from build123d import *

# Parameters (mm, degrees)
SKETCH_1_W          = 553
SKETCH_1_H          = 333
EXTRUDE_1_DEPTH     = 56
FILLET_1_SIZE       = 40
FILLET_1_SIZE_2     = 150
SKETCH_2_W          = 526
SKETCH_2_H          = 298
CUT_EXTRUDE_1_DEPTH = 1
SKETCH_3_W          = 90
SKETCH_3_H          = 7.88506372
EXTRUDE_2_DEPTH     = 3


with BuildPart() as part:
    # Эскиз1 → Бобышка-Вытянуть1 (new body)
    with BuildSketch(Plane.XY):
        with Locations((219.863599641, -140.079802513)):
            Rectangle(SKETCH_1_W, SKETCH_1_H)
    extrude(amount=-EXTRUDE_1_DEPTH)

    # Скругление1
    # an asymmetric fillet: 150, 40 mm, written as the material it takes off along each edge
    with BuildSketch(Plane(origin=(496.363599641, -306.579802513, -56), x_dir=(0, 0, 1), z_dir=(-1, 0, 0)), Plane(origin=(-56.636400359, 26.420197487, -56), x_dir=(0, 0, 1), z_dir=(1, 0, 0))) as fillet_1_piece_1:
        with BuildLine():
            Bezier((FILLET_1_SIZE, 0), (0, 0), (0, FILLET_1_SIZE_2), weights=[1, 0.707106781, 1])
            Line((0, FILLET_1_SIZE_2), (-3, 150))
            Line((-3, 150), (-3, -3))
            Line((-3, -3), (40, -3))
            Line((40, -3), (FILLET_1_SIZE, 0))
        make_face()
    extrude(amount=553, mode=Mode.SUBTRACT)
    with BuildSketch(Plane(origin=(-56.636400359, -306.579802513, -56), x_dir=(0, 0, 1), z_dir=(0, 1, 0)), Plane(origin=(496.363599641, 26.420197487, -56), x_dir=(0, 0, 1), z_dir=(0, -1, 0))) as fillet_1_piece_2:
        with BuildLine():
            Bezier((FILLET_1_SIZE, 0), (0, 0), (0, FILLET_1_SIZE_2), weights=[1, 0.707106781, 1])
            Line((0, FILLET_1_SIZE_2), (-3, 150))
            Line((-3, 150), (-3, -3))
            Line((-3, -3), (40, -3))
            Line((40, -3), (FILLET_1_SIZE, 0))
        make_face()
    extrude(amount=333, mode=Mode.SUBTRACT)
    with BuildSketch(Plane(origin=(496.363599641, 26.420197487, -56), x_dir=(0, 0, 1), z_dir=(0, -1, 0))) as fillet_1_piece_3a_section:
        with BuildLine():
            Bezier((FILLET_1_SIZE, 0), (0, 0), (0, FILLET_1_SIZE_2), weights=[1, 0.707106781, 1])
            Line((0, FILLET_1_SIZE_2), (-3, 150))
            Line((-3, 150), (-3, -3))
            Line((-3, -3), (40, -3))
            Line((40, -3), (FILLET_1_SIZE, 0))
        make_face()
    fillet_1_piece_3a = extrude(amount=708, mode=Mode.PRIVATE)
    fillet_1_piece_3a = split(fillet_1_piece_3a, bisect_by=Plane(origin=(455.274079594, -306.579802513, -48.919820082), z_dir=(0, -1, 0)), keep=Keep.TOP, mode=Mode.PRIVATE)
    with BuildSketch(Plane(origin=(871.363599641, -306.579802513, -56), x_dir=(0, 0, 1), z_dir=(-1, 0, 0))) as fillet_1_piece_3b_section:
        with BuildLine():
            Bezier((FILLET_1_SIZE, 0), (0, 0), (0, FILLET_1_SIZE_2), weights=[1, 0.707106781, 1])
            Line((0, FILLET_1_SIZE_2), (-3, 150))
            Line((-3, 150), (-3, -3))
            Line((-3, -3), (40, -3))
            Line((40, -3), (FILLET_1_SIZE, 0))
        make_face()
    fillet_1_piece_3b = extrude(amount=928, mode=Mode.PRIVATE)
    fillet_1_piece_3b = split(fillet_1_piece_3b, bisect_by=Plane(origin=(496.363599641, -265.490295874, -48.919826396), z_dir=(1, 0, 0)), keep=Keep.TOP, mode=Mode.PRIVATE)
    fillet_1_piece_3 = fillet_1_piece_3a & fillet_1_piece_3b
    add(fillet_1_piece_3, mode=Mode.SUBTRACT)
    with BuildSketch(Plane(origin=(496.363599641, -306.579802513, -56), x_dir=(0, 0, 1), z_dir=(-1, 0, 0))) as fillet_1_piece_4a_section:
        with BuildLine():
            Bezier((FILLET_1_SIZE, 0), (0, 0), (0, FILLET_1_SIZE_2), weights=[1, 0.707106781, 1])
            Line((0, FILLET_1_SIZE_2), (-3, 150))
            Line((-3, 150), (-3, -3))
            Line((-3, -3), (40, -3))
            Line((40, -3), (FILLET_1_SIZE, 0))
        make_face()
    fillet_1_piece_4a = extrude(amount=928, mode=Mode.PRIVATE)
    fillet_1_piece_4a = split(fillet_1_piece_4a, bisect_by=Plane(origin=(-56.636400359, -265.49028305, -48.919819953), z_dir=(-1, 0, 0)), keep=Keep.TOP, mode=Mode.PRIVATE)
    with BuildSketch(Plane(origin=(-56.636400359, -681.579802513, -56), x_dir=(0, 0, 1), z_dir=(0, 1, 0))) as fillet_1_piece_4b_section:
        with BuildLine():
            Bezier((FILLET_1_SIZE, 0), (0, 0), (0, FILLET_1_SIZE_2), weights=[1, 0.707106781, 1])
            Line((0, FILLET_1_SIZE_2), (-3, 150))
            Line((-3, 150), (-3, -3))
            Line((-3, -3), (40, -3))
            Line((40, -3), (FILLET_1_SIZE, 0))
        make_face()
    fillet_1_piece_4b = extrude(amount=708, mode=Mode.PRIVATE)
    fillet_1_piece_4b = split(fillet_1_piece_4b, bisect_by=Plane(origin=(-15.546893136, -306.579802513, -48.919826525), z_dir=(0, -1, 0)), keep=Keep.TOP, mode=Mode.PRIVATE)
    fillet_1_piece_4 = fillet_1_piece_4a & fillet_1_piece_4b
    add(fillet_1_piece_4, mode=Mode.SUBTRACT)
    with BuildSketch(Plane(origin=(-431.636400359, 26.420197487, -56), x_dir=(0, 0, 1), z_dir=(1, 0, 0))) as fillet_1_piece_5a_section:
        with BuildLine():
            Bezier((FILLET_1_SIZE, 0), (0, 0), (0, FILLET_1_SIZE_2), weights=[1, 0.707106781, 1])
            Line((0, FILLET_1_SIZE_2), (-3, 150))
            Line((-3, 150), (-3, -3))
            Line((-3, -3), (40, -3))
            Line((40, -3), (FILLET_1_SIZE, 0))
        make_face()
    fillet_1_piece_5a = extrude(amount=928, mode=Mode.PRIVATE)
    fillet_1_piece_5a = split(fillet_1_piece_5a, bisect_by=Plane(origin=(-56.636400359, -14.669309261, -48.919826397), z_dir=(-1, 0, 0)), keep=Keep.TOP, mode=Mode.PRIVATE)
    with BuildSketch(Plane(origin=(-56.636400359, -306.579802513, -56), x_dir=(0, 0, 1), z_dir=(0, 1, 0))) as fillet_1_piece_5b_section:
        with BuildLine():
            Bezier((FILLET_1_SIZE, 0), (0, 0), (0, FILLET_1_SIZE_2), weights=[1, 0.707106781, 1])
            Line((0, FILLET_1_SIZE_2), (-3, 150))
            Line((-3, 150), (-3, -3))
            Line((-3, -3), (40, -3))
            Line((40, -3), (FILLET_1_SIZE, 0))
        make_face()
    fillet_1_piece_5b = extrude(amount=708, mode=Mode.PRIVATE)
    fillet_1_piece_5b = split(fillet_1_piece_5b, bisect_by=Plane(origin=(-15.546880312, 26.420197487, -48.919820082), z_dir=(0, 1, 0)), keep=Keep.TOP, mode=Mode.PRIVATE)
    fillet_1_piece_5 = fillet_1_piece_5a & fillet_1_piece_5b
    add(fillet_1_piece_5, mode=Mode.SUBTRACT)
    with BuildSketch(Plane(origin=(-56.636400359, 26.420197487, -56), x_dir=(0, 0, 1), z_dir=(1, 0, 0))) as fillet_1_piece_6a_section:
        with BuildLine():
            Bezier((FILLET_1_SIZE, 0), (0, 0), (0, FILLET_1_SIZE_2), weights=[1, 0.707106781, 1])
            Line((0, FILLET_1_SIZE_2), (-3, 150))
            Line((-3, 150), (-3, -3))
            Line((-3, -3), (40, -3))
            Line((40, -3), (FILLET_1_SIZE, 0))
        make_face()
    fillet_1_piece_6a = extrude(amount=928, mode=Mode.PRIVATE)
    fillet_1_piece_6a = split(fillet_1_piece_6a, bisect_by=Plane(origin=(496.363599641, -14.669322085, -48.919819954), z_dir=(1, 0, 0)), keep=Keep.TOP, mode=Mode.PRIVATE)
    with BuildSketch(Plane(origin=(496.363599641, 401.420197487, -56), x_dir=(0, 0, 1), z_dir=(0, -1, 0))) as fillet_1_piece_6b_section:
        with BuildLine():
            Bezier((FILLET_1_SIZE, 0), (0, 0), (0, FILLET_1_SIZE_2), weights=[1, 0.707106781, 1])
            Line((0, FILLET_1_SIZE_2), (-3, 150))
            Line((-3, 150), (-3, -3))
            Line((-3, -3), (40, -3))
            Line((40, -3), (FILLET_1_SIZE, 0))
        make_face()
    fillet_1_piece_6b = extrude(amount=708, mode=Mode.PRIVATE)
    fillet_1_piece_6b = split(fillet_1_piece_6b, bisect_by=Plane(origin=(455.274092417, 26.420197487, -48.919826525), z_dir=(0, 1, 0)), keep=Keep.TOP, mode=Mode.PRIVATE)
    fillet_1_piece_6 = fillet_1_piece_6a & fillet_1_piece_6b
    add(fillet_1_piece_6, mode=Mode.SUBTRACT)

    # Эскиз2 → Вырез-Вытянуть1 (cut)
    with BuildSketch(Plane.XY):
        with Locations((219.863599641, -134.579802513)):
            Rectangle(SKETCH_2_W, SKETCH_2_H)
    extrude(amount=-CUT_EXTRUDE_1_DEPTH, mode=Mode.SUBTRACT)

    # Эскиз3 → Бобышка-Вытянуть2 (add)
    with BuildSketch(Plane.XZ.offset(306.579802513)):
        with Locations((416.363599641, -8.14121692)):
            Rectangle(SKETCH_3_W, SKETCH_3_H)
    extrude(amount=EXTRUDE_2_DEPTH)


solid = part.part
Check sheet for the modelled part. Datum: model origin and axes. Units: mm. Round coordinates to 2 decimals unless told otherwise and drop trailing zeros.
1. Mould release check, pull along X, two halves, no side actions. Record for faces 1 (the flat face through (216, 26.42, -8)), 2 (the flat face through (216, -132, -1)), 3 (the flat face through (496.364, -142, -8)): released by +X, released by -X, zero draft, split by the parting line, or undercut.
2. Scan lines: probe 1 along Y at (x, z) = (76, -7); probe 2 along Z at (x, y) = (397.5, -193.5); probe 3 along Z at (x, y) = (385, -281). Record each from-to range of solid material in increasing order.
3. Gauge pin test, flat ends, axial feed: pin 1 Ø2.5 at (x, y) = (414, -308.5) entering from +Z; pin 2 Ø1.5 at (x, y) = (192, -18.5) entering from +Z; pin 3 Ø0.9 at (x, y) = (432.5, -308.5) entering from -Z; pin 4 Ø2.5 at (y, z) = (-307.5, -7) entering from +X. Record the tip position at first contact, or that the pin passes through.
Recorded:
1. face 1: zero draft
1. face 2: undercut
1. face 3: released by +X
2. probe 1: y = -306.58 to 26.42
2. probe 2: z = -53.6 to -1
2. probe 3: z = -38.34 to -1
3. pin 1: stops at z = -4.2
3. pin 2: stops at z = -1
3. pin 3: stops at z = -12.08
3. pin 4: stops at x = 496.36
